from build123d import *

# Parameters (mm, degrees)
F0_R     = 3.3
F1_DEPTH = 4
F2_R     = 1


with BuildPart() as f1:
    # F0 (on Front) → F1 (new body)
    with BuildSketch(Plane.XZ):
        with BuildLine():
            ThreePointArc((34.044412, 89.907971), (40.707021, 94.393881), (36.938175, 101.486803))
            ThreePointArc((36.938175, 101.486803), (0, 108), (-36.938175, 101.486803))
            ThreePointArc((-36.938175, 101.486803), (-40.707021, 94.393881), (-34.044412, 89.907971))
            ThreePointArc((-34.044412, 89.907971), (-32.023131, 89.475058), (-30.761711, 87.837435))
            Line((-30.761711, 87.837435), (-29.240737, 82.999875))
            ThreePointArc((-29.240737, 82.999875), (-21.913547, 79.017697), (-17.683893, 86.204872))
            Line((-17.683893, 86.204872), (-18.821651, 90.927144))
            ThreePointArc((-18.821651, 90.927144), (-18.41244, 93.277047), (-16.418177, 94.585641))
            ThreePointArc((-16.418177, 94.585641), (-12.945689, 95.123126), (-9.455857, 95.533171))
            ThreePointArc((-9.455857, 95.533171), (-7.184419, 94.805114), (-6.162106, 92.650032))
            Line((-6.162106, 92.650032), (-5.996512, 87.795455))
            ThreePointArc((-5.996512, 87.795455), (0, 82), (5.996512, 87.795455))
            Line((5.996512, 87.795455), (6.162106, 92.650032))
            ThreePointArc((6.162106, 92.650032), (7.184419, 94.805114), (9.455857, 95.533171))
            ThreePointArc((9.455857, 95.533171), (12.945689, 95.123126), (16.418177, 94.585641))
            ThreePointArc((16.418177, 94.585641), (18.41244, 93.277047), (18.821651, 90.927144))
            Line((18.821651, 90.927144), (17.683893, 86.204872))
            ThreePointArc((17.683893, 86.204872), (21.913547, 79.017697), (29.240737, 82.999875))
            Line((29.240737, 82.999875), (30.761711, 87.837435))
            ThreePointArc((30.761711, 87.837435), (32.023131, 89.475058), (34.044412, 89.907971))
        make_face()
        with Locations((-23.516977, 84.79948)):
            Circle(F0_R, mode=Mode.SUBTRACT)
        with Locations((0, 88)):
            Circle(F0_R, mode=Mode.SUBTRACT)
        with Locations((23.516977, 84.79948)):
            Circle(F0_R, mode=Mode.SUBTRACT)
        with BuildLine():
            ThreePointArc((-35.912115, 98.667725), (0, 105), (35.912115, 98.667725))
            ThreePointArc((35.912115, 98.667725), (37.705132, 94.822587), (33.859994, 93.029569))
            ThreePointArc((33.859994, 93.029569), (0, 99), (-33.859994, 93.029569))
            ThreePointArc((-33.859994, 93.029569), (-37.705132, 94.822587), (-35.912115, 98.667725))
        make_face(mode=Mode.SUBTRACT)
    extrude(amount=F1_DEPTH)

    # F2
    f2_edges = [f1.edges().sort_by_distance(p)[0] for p in [
        (0, -4, 108),
    ]]
    fillet(f2_edges, radius=F2_R)


solid = f1.part
CAD build for the part. Positions are in the model's coordinates, mm. A direction names the side the tool comes from. Round coordinates to 2 decimals unless told otherwise and drop trailing zeros. Loops run counter-clockwise (first coordinate to the right, second up) from the corner with the lowest first, then second, coordinate; pieces in that order, holes last. Notation, with made-up numbers: M -15,-26 L 31,-26 A18 cw 31,-22 Z; hole C 14.25,1 d7. An arc over 180 degrees is marked long. One line per question, with ' | ' between items. Start each with the question number.
Item 1: Cut at A-A, the plane x = 0. Write the cut outline in (y, z), plus the area to 3 significant figures.
Item 2: Which spindle directions (+Z, -Z, +X, -X, +Y, -Y) get a long thin tool onto all of the face, cutting with end or side? Do faces 4 (the cylindrical face through (-29.72, -3.7, 85.47)), 5 (the cylindrical face through (0, -2, 99)), 6 (the cylindrical face through (12.9, -1.48, 95.13)). Say none if no direction does.
Item 3: Cut at C-C, the plane x = -23. State how many separate pieces and enclosed holes the cut face has, plus the area to 3 significant figures.
Item 4: Two-plate mould, pull along Z, no slides. Class faces 1 (the cylindrical face through (0.5, -1.5, 108)), 2 (the cylindrical face through (-7.21, -1.479, 94.828)), 3 (the cylindrical face through (25.04, -1.97, 81.87)): pulls with the +Z half, pulls with the -Z half, needs draft (parallel to the pull), parting line crosses it, or undercut.
Item 5: Wall check: line 1 (X direction, y = -1.1, z = 84); line 2 (X direction, y = -0.65, z = 88.5); line 3 (Z direction, x = -2.5, y = -1.5). Give the ranges that are in metal, low to high.
Item 6: Pin check, flat tips, straight feed: pin 1 Ø5.5 at (x, z) = (0, 88) entering from -Y; pin 2 Ø2 at (x, z) = (6.5, 88) entering from -Y; pin 3 Ø1 at (x, y) = (-16, -3.5) entering from +Z; pin 4 Ø1.5 at (x, y) = (-20.5, -1.5) entering from -Z. Stop position of each tip, or through.
Item 7: Cut at B-B, the plane y = -1.65. Write the cut outline in (x, z), plus the area to 3 significant figures.
Responses:
1) outline: M -4,83 A1 ccw -3,82 L 0,82 L 0,84.7 L -4,84.7 Z; M -4,91.3 L 0,91.3 L 0,99 L -4,99 Z; M -4,105 L 0,105 L 0,108 L -3,108 A1 ccw -4,107 Z | area: 53.2 mm²
2) face 4: -Z, -X, -Y | face 5: +Y, -Y | face 6: -Z, +Y, -Y
3) separate pieces: 3 | enclosed holes: 0 | area: 55.7 mm²
4) face 1: pulls with the +Z half | face 2: pulls with the -Z half | face 3: undercut
5) line 1: x = -29.56 to -26.72, -20.32 to -17.57, -4.47 to 4.47, 17.57 to 20.32, 26.72 to 29.56 | line 2: x = -31.06 to -18.24, -6.02 to -3.26, 3.26 to 6.02, 18.24 to 31.06 | line 3: z = 82.55 to 85.85, 90.15 to 98.97, 104.97 to 107.97
6) pin 1: passes through | pin 2: stops at y = -3.87 | pin 3: stops at z = 106.85 | pin 4: stops at z = 79.24
7) outline: M -36.94,101.49 A6 ccw -34.04,89.91 A3 cw -30.76,87.84 L -29.24,83 A6 ccw -17.68,86.2 L -18.82,90.93 A3 cw -16.42,94.59 A96 cw -9.46,95.53 A3 cw -6.16,92.65 L -6,87.8 A6 ccw 6,87.8 L 6.16,92.65 A3 cw 9.46,95.53 A96 cw 16.42,94.59 A3 cw 18.82,90.93 L 17.68,86.2 A6 ccw 29.24,83 L 30.76,87.84 A3 cw 34.04,89.91 A6 ccw 36.94,101.49 A108 ccw Z; hole M -35.91,98.67 A3 ccw -33.86,93.03 A99 cw 33.86,93.03 A3 ccw 35.91,98.67 A105 ccw Z; hole C -23.52,84.8 d6.6; hole C 0,88 d6.6; hole C 23.52,84.8 d6.6 | area: 883 mm²
